```python
from build123d import *

# Parameters (mm, degrees)
F0_R     = 3.175
F1_DEPTH = 3.048


with BuildPart() as f1:
    # F0 (on Front) → F1 (new body)
    with BuildSketch(Plane.XZ):
        with BuildLine():
            ThreePointArc((-9.525, 114.3), (-6.7351920908, 107.5648079092), (0, 104.775))
            ThreePointArc((0, 104.775), (6.7351920908, 107.5648079092), (9.525, 114.3))
            ThreePointArc((9.525, 114.3), (9.5084619879, 114.8610486832), (9.4589053806, 115.4201490977))
            ThreePointArc((9.4589053806, 115.4201490977), (-0.5610486832, 123.8084619879), (-9.525, 114.3))
        make_face()
        with BuildLine():
            ThreePointArc((3.175, 114.3), (2.2450640303, 112.0549359697), (0, 111.125))
            ThreePointArc((0, 111.125), (-2.2450640303, 116.5450640303), (3.175, 114.3))
        make_face(mode=Mode.SUBTRACT)
        with BuildLine():
            ThreePointArc((9.525, 114.3), (6.7351920908, 107.5648079092), (0, 104.775))
            Line((0, 104.775), (0, 79.375))
            ThreePointArc((0, 79.375), (9.1908363712, 76.4438847259), (14.9877324754, 68.7329246359))
            Line((14.9877324754, 68.7329246359), (9.4589053806, 115.4201490977))
            ThreePointArc((9.4589053806, 115.4201490977), (9.5084619879, 114.8610486832), (9.525, 114.3))
        make_face()
        with BuildLine():
            Line((0, 79.375), (0, 104.775))
            ThreePointArc((0, 104.775), (-6.7351920908, 107.5648079092), (-9.525, 114.3))
            Line((-9.525, 114.3), (-15.7474569047, 65.5082893304))
            ThreePointArc((-15.7474569047, 65.5082893304), (-10.4912828548, 75.4142187767), (0, 79.375))
        make_face()
        with Locations((-5.5348160677, 97.4346920848)):
            Circle(F0_R, mode=Mode.SUBTRACT)
        with BuildLine():
            ThreePointArc((14.9877324754, 68.7329246359), (9.1908363712, 76.4438847259), (0, 79.375))
            Line((0, 79.375), (0, 65.0875))
            ThreePointArc((0, 65.0875), (1.1225320151, 64.6225320151), (1.5875, 63.5))
            ThreePointArc((1.5875, 63.5), (1.1225320151, 62.3774679849), (0, 61.9125))
            Line((0, 61.9125), (0, 47.625))
            ThreePointArc((0, 47.625), (10.6492737428, 51.7267849017), (15.7954255641, 61.9125))
            Line((15.7954255641, 61.9125), (14.9877324754, 68.7329246359))
        make_face()
        with BuildLine():
            Line((0, 65.0875), (0, 79.375))
            ThreePointArc((0, 79.375), (-10.4912828548, 75.4142187767), (-15.7474569047, 65.5082893304))
            ThreePointArc((-15.7474569047, 65.5082893304), (-15.8735876171, 63.7117573215), (-15.7954255641, 61.9125))
            ThreePointArc((-15.7954255641, 61.9125), (-10.6492737428, 51.7267849017), (0, 47.625))
            Line((0, 47.625), (0, 61.9125))
            ThreePointArc((0, 61.9125), (-1.5875, 63.5), (0, 65.0875))
        make_face()
        with BuildLine():
            Line((11.3408358685, 17.5898921545), (15.7954255641, 61.9125))
            ThreePointArc((15.7954255641, 61.9125), (10.6492737428, 51.7267849017), (0, 47.625))
            Line((0, 47.625), (0, 9.525))
            ThreePointArc((0, 9.525), (6.7351920908, 6.7351920908), (9.525, 0))
            Line((9.525, 0), (36.5125, 0))
            ThreePointArc((36.5125, 0), (38.9380895153, 5.7116327839), (44.7324052746, 7.9324746146))
            Line((44.7324052746, 7.9324746146), (18.968327868, 8.8497055806))
            ThreePointArc((18.968327868, 8.8497055806), (13.2612039825, 11.5674628959), (11.3408358685, 17.5898921545))
        make_face()
        with BuildLine():
            ThreePointArc((0, 47.625), (-10.6492737428, 51.7267849017), (-15.7954255641, 61.9125))
            Line((-15.7954255641, 61.9125), (-9.4772553384, -0.9525))
            ThreePointArc((-9.4772553384, -0.9525), (-7.063929059, 6.3895642457), (0, 9.525))
            Line((0, 9.525), (0, 47.625))
        make_face()
        with BuildLine():
            ThreePointArc((0, 9.525), (-7.063929059, 6.3895642457), (-9.4772553384, -0.9525))
            ThreePointArc((-9.4772553384, -0.9525), (-6.3895642457, -7.063929059), (0, -9.525))
            Line((0, -9.525), (0.6773435479, -9.500885786))
            ThreePointArc((0.6773435479, -9.500885786), (6.9705567315, -6.4912990883), (9.525, 0))
            Line((9.525, 0), (4.8608528189, 0))
            ThreePointArc((4.8608528189, 0), (-3.4371419906, -3.4371419906), (0, 4.8608528189))
            Line((0, 4.8608528189), (0, 9.525))
        make_face()
        with BuildLine():
            ThreePointArc((9.525, 0), (6.7351920908, 6.7351920908), (0, 9.525))
            Line((0, 9.525), (0, 4.8608528189))
            ThreePointArc((0, 4.8608528189), (3.4371419906, 3.4371419906), (4.8608528189, 0))
            Line((4.8608528189, 0), (9.525, 0))
        make_face()
        with BuildLine():
            Line((36.5125, 0), (9.525, 0))
            ThreePointArc((9.525, 0), (6.9705567315, -6.4912990883), (0.6773435479, -9.500885786))
            Line((0.6773435479, -9.500885786), (44.7324052746, -7.9324746146))
            ThreePointArc((44.7324052746, -7.9324746146), (38.9380895153, -5.7116327839), (36.5125, 0))
        make_face()
        with BuildLine():
            ThreePointArc((52.3875, 0), (50.1616327839, 5.5119104847), (44.7324052746, 7.9324746146))
            ThreePointArc((44.7324052746, 7.9324746146), (38.9380895153, 5.7116327839), (36.5125, 0))
            Line((36.5125, 0), (40.655729, 0))
            ThreePointArc((40.655729, 0), (44.45, 3.794271), (48.244271, 0))
            Line((48.244271, 0), (52.3875, 0))
        make_face()
        with BuildLine():
            Line((40.655729, 0), (36.5125, 0))
            ThreePointArc((36.5125, 0), (38.9380895153, -5.7116327839), (44.7324052746, -7.9324746146))
            ThreePointArc((44.7324052746, -7.9324746146), (50.1616327839, -5.5119104847), (52.3875, 0))
            Line((52.3875, 0), (48.244271, 0))
            ThreePointArc((48.244271, 0), (44.45, -3.794271), (40.655729, 0))
        make_face()
    extrude(amount=F1_DEPTH)


solid = f1.part
```
Could you check a few things on this model? Use its own coordinates, in mm. A direction names the side the tool comes from. Give positions to 0.01 mm unless a question says otherwise; leave off trailing zeros. Loops run counter-clockwise (first coordinate to the right, second up) from the corner with the lowest first, then second, coordinate; pieces in that order, holes last. Notation, with made-up numbers: (72.25, -34.75) -> (88.25, -34.75) arc R5 ccw to (88.25, -30.75) -> close; hole circle Ø3 at (-17, 44). An arc over 180 degrees is marked (long way). Put each result on its own line as item: value.
(1) I'm going to push a flat-ended pin straight in: pin 1 Ø10 at (x, z) = (0, 114.3) entering from -Y. Where does the tip first touch, or does it pass through?
Computed:
pin 1: y = -3.05
(2) For faces 1 (the face through (13.32, -1.5, 11.5)), 2 (the face through (3, 0, 43)), which set-ups out of +Z, -Z, +X, -X, +Y, -Y let a thin tool reach every point of the face, with its end or its side?
Computed:
face 1: +X, +Y, -Y
face 2: +Z, -Z, +X, -X, +Y
(3) Please list where these lines run through material, in increasing order: probe 1 along Z at (x, y) = (-2, -2.8); probe 2 along Z at (x, y) = (2.5, -1.85); probe 3 along X at (y, z) = (-1.6, -2.5). Write a range as [from, to].
Computed:
probe 1: [-9.31, -4.43], [4.43, 111.83], [116.77, 123.61]
probe 2: [-9.44, -4.17], [4.17, 112.34], [116.26, 123.49]
probe 3: [-9.19, -4.17], [4.17, 41.6], [47.3, 51.98]
(4) Thinking about a two-plate mould opening in X: for faces 3 (the face through (-12.6, -1.5, 90.2)), 4 (the face through (40.66, -1.5, -0.17)), 5 (the face through (-0.36, -1.5, 123.82)), which applies, pulls with the +X half, pulls with the -X half, needs draft (parallel to the pull), parting line crosses it, or undercut?
Computed:
face 3: pulls with the -X half
face 4: undercut
face 5: parting line crosses it
(5) Imagine slicing it at C-C on z = 80. Write out the boundary of the cut face in (x, y), plus the area to 3 significant figures.
Computed:
outline: (-13.9, -3.05) -> (13.65, -3.05) -> (13.65, 0) -> (-13.9, 0) -> close
area: 84.0 mm^2
(6) Imagine slicing it at A-A on y = -2.4. State how many separate pieces and enclosed holes the cut face has, plus the area to 3 significant figures.
Computed:
separate pieces: 1
enclosed holes: 5
area: 3,730 mm^2
(7) Imagine slicing it at B-B on x = 35. Write out the boundary of the cut face in (y, z), plus the area to 3 significant figures.
Computed:
outline: (-3.05, -8.28) -> (0, -8.28) -> (0, 8.28) -> (-3.05, 8.28) -> close
area: 50.5 mm^2
